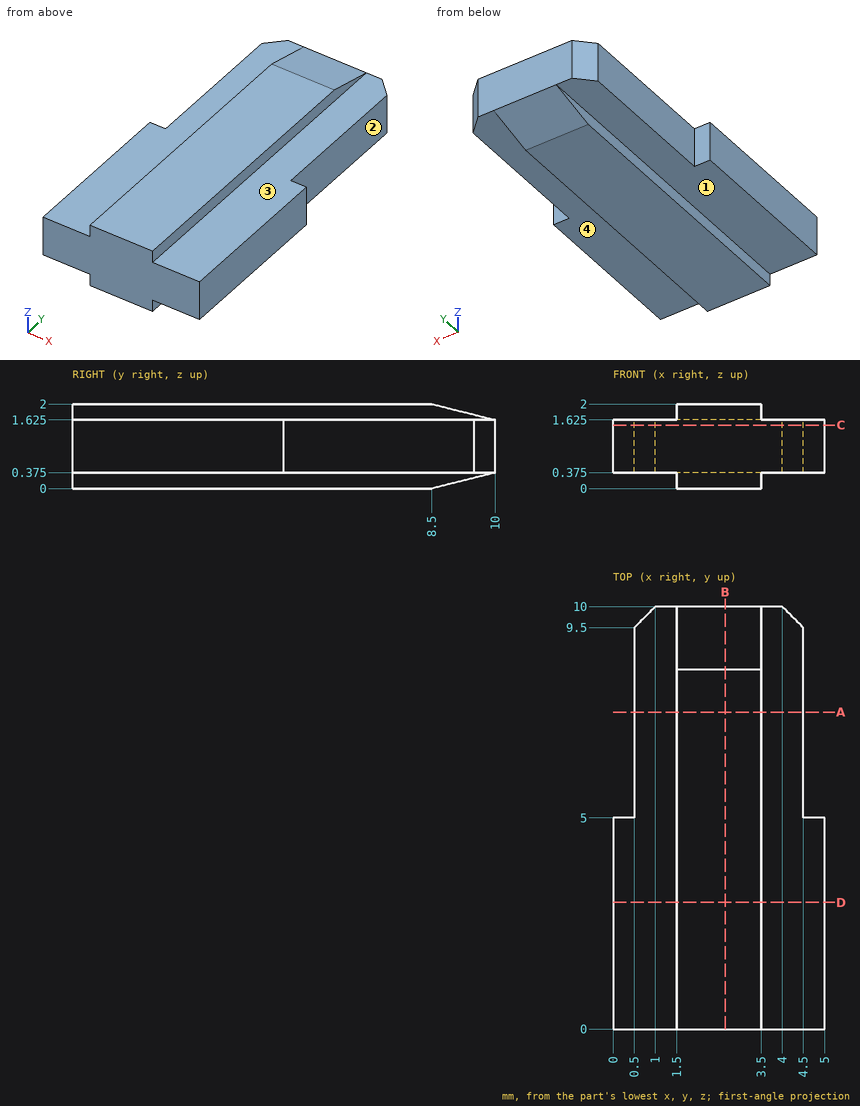
Check sheet for the drawn part. Datum: minimum x, y, z corner. Units: mm. A direction names the side the tool comes from. Give positions to 0.01 mm unless a question says otherwise; leave off trailing zeros. Order: outer loops, then holes, each group sorted by start corner. A loop starts at its lowest first (then second) coordinate and runs counter-clockwise, first axis right, second up. Notation, with made-up numbers: (7, -28.75) - (16, -28.75) arc R4 cw to (16, -23.75) - close; hole circle Ø7 at (-12, 11). An arc over 180 degrees is marked (long way). Write item = value, one per line. Start each with the question number.
1) Section check C-C (z = 1.5). Enter the section's corners in (x, y).
2) Section check D-D (y = 3). Enter the section's corners in (x, z) (3 decimals), then the cut area to 3 significant figures.
3) Access from +Z, -Z, +X, -X, +Y, -Y to the whole of each face (thin tool, end or side, straight path). Record for the marked faces 1, 2, 3 and 4.
4) Section check B-B (x = 2.65). Enter the section's corners in (y, z) (3 decimals).
5) Gauge pin test, flat end, axial feed: pin 1 Ø0.8 at (x, y) = (1, 4) entering from -Z (3 decimals). Record the tip position at first contact, or that the pin passes through.
6) Scan lines: L1, parallel to X at y = 4.25, z = 1.75; L2, parallel to Z at x = 0.2, y = 4 (3 decimals); L3, parallel to X at y = 7, z = 1.5. Record each from-to range of solid material in increasing order.
7) Section check A-A (y = 7.5). Enter the section's corners in (x, z) (3 decimals).
Geometry check:
q1.outline = (0, 0) - (5, 0) - (5, 5) - (4.5, 5) - (4.5, 9.5) - (4, 10) - (1, 10) - (0.5, 9.5) - (0.5, 5) - (0, 5) - close
q2.outline = (0, 0.375) - (1.5, 0.375) - (1.5, 0) - (3.5, 0) - (3.5, 0.375) - (5, 0.375) - (5, 1.625) - (3.5, 1.625) - (3.5, 2) - (1.5, 2) - (1.5, 1.625) - (0, 1.625) - close
q2.area = 7.75 mm2
q3.face_1 = -Z, -X, +Y, -Y
q3.face_2 = +Z, -Z, +X, +Y
q3.face_3 = +Z, +X, +Y, -Y
q3.face_4 = -Z, +X, +Y, -Y
q4.outline = (0, 0) - (8.5, 0) - (10, 0.375) - (10, 1.625) - (8.5, 2) - (0, 2) - close
q5.pin_1 = 0.375
q6.L1 = 1.5 to 3.5
q6.L2 = 0.375 to 1.625
q6.L3 = 0.5 to 4.5
q7.outline = (0.5, 0.375) - (1.5, 0.375) - (1.5, 0) - (3.5, 0) - (3.5, 0.375) - (4.5, 0.375) - (4.5, 1.625) - (3.5, 1.625) - (3.5, 2) - (1.5, 2) - (1.5, 1.625) - (0.5, 1.625) - close
